Autodesk Inventor part; units mm, degrees
ref_plane "YZ Plane" through (0, 0, 0) normal (1, 0, 0) x (0, 1, 0)
ref_plane "XZ Plane" through (0, 0, 0) normal (0, 1, 0) x (-1, 0, 0)
ref_plane "XY Plane" through (0, 0, 0) normal (0, 0, 1) x (1, 0, 0)
sketch "Sketch1" plane through (0, 0, 0) normal (0, 1, 0) x (-1, 0, 0)
  circle A0 centre (0, 0) radius 7.5
  dimension "d0" = 15
extrude "Extrusion1" add sketch "Sketch1" along normal blind 12
sketch "Sketch2" plane through (0, 0, 0) normal (0, -1, 0) x (1, 0, 0)
  circle A0 centre (0, 0) radius 7.5
  line L0 (-2.5206, -7.0638) -> (2.5206, -7.0638)
  line L1 (2.5206, -7.0638) -> (2.5206, 7.0638)
  line L2 (2.5206, 7.0638) -> (-2.5206, 7.0638)
  line L3 (-2.5206, 7.0638) -> (-2.5206, -7.0638)
  line L4 (-2.5206, -7.0638) -> (2.5206, 7.0638) construction
  line L5 (2.5206, -7.0638) -> (-2.5206, 7.0638) construction
extrude "Extrusion2" add sketch "Sketch2" along normal blind 7 contours L1 L0 L3 L2
thread "Thread1"
properties part number "voet"
Source: CAD feature listing. Evaluate the final solid. Frame: model axes, mm. A direction names the side the tool comes from. Coordinates: 2 decimals unless noted, no trailing zeros. Loops run counter-clockwise (first coordinate to the right, second up) from the corner with the lowest first, then second, coordinate; pieces in that order, holes last. Notation, with made-up numbers: (5.5, -37) - (23.5, -37) arc R13 ccw to (23.5, -27) - close; hole circle Ø8 at (-1, 86). An arc over 180 degrees is marked (long way). Return JSON: item names as keys, results as strings.
Q1. Section B-B, the plane z = 2.5. Return loops of the section in (x, y).
Results:
{"outline": "(-7.07, 0) - (-2.52, 0) - (-2.52, -7) - (2.52, -7) - (2.52, 0) - (7.07, 0) - (7.07, 12) - (-7.07, 12) - close"}
Q2. Section C-C, the plane y = 3.75. Return loops of the section in (x, z).
Results:
{"outline": "circle Ø15 at (0, 0)"}
Q3. Material intervals for line 1 along Y through (x, z) = (-4.5, 1.25); line 2 along Z through (x, y) = (1, -1.25); line 3 along X through (y, z) = (1, -2.5), sorted ascending.
Results:
{"line 1": "0 to 12", "line 2": "-7.06 to 7.06", "line 3": "-7.07 to 7.07"}
Q4. Section D-D, the plane y = -4.5. Return loops of the section in (x, z).
Results:
{"outline": "(-2.52, -7.06) - (2.52, -7.06) - (2.52, 7.06) - (-2.52, 7.06) - close"}
Q5. Mould query, pull axis X, two halves, no side actions, for faces 5 (the flat face through (-2.521, -3, 0)), 6 (the flat face through (0, -3, -7.064)), 7 (the cylindrical face through (7.493, 5.916, -0.33)). Classes: released by +X, released by -X, zero draft, split by the parting line, or undercut.
Results:
{"face 5": "released by -X", "face 6": "zero draft", "face 7": "split by the parting line"}
Q6. Access query for faces 1 (the flat face through (4, 0, 0)), 2 (the flat face through (-4, 0, 0)), 3 (the flat face through (0, -3, 7.064)), 4 (the flat face through (0, -7, 0)). Directions: +Z, -Z, +X, -X, +Y, -Y. A direction counts if a zero-diameter tool reaches every point of the face in a straight line with its end or side. Return the directions, or none.
Results:
{"face 1": "+Z, -Z, +X, -Y", "face 2": "+Z, -Z, -X, -Y", "face 3": "+Z, +X, -X, -Y", "face 4": "+Z, -Z, +X, -X, -Y"}
Q7. Section A-A, the plane x = 0. Return loops of the section in (y, z), plus the area to 3 significant figures.
Results:
{"outline": "(-7, -7.06) - (0, -7.06) - (0, -7.5) - (12, -7.5) - (12, 7.5) - (0, 7.5) - (0, 7.06) - (-7, 7.06) - close", "area": "279 mm2"}
Q8. Contact query for flat-ended pins moving along their axis: P1, Ø1.5, axis at x = -0.5, y = -4.5, coming from the +Z side; P2, Ø5.5, axis at y = -3.5, z = 0, coming from the +X side; P3, Ø0.5, axis at x = -1, z = 7.5, coming from the -Y side. Output: stop coordinate, or through.
Results:
{"P1": "z = 7.06", "P2": "x = 2.52", "P3": "y = 0"}
